```python
from build123d import *

# Parameters (mm, degrees)
SKETCH_W        = 130
SKETCH_H        = 40
SKETCH_R        = 8.5
PAD_DEPTH       = 3
SKETCH001_R     = 1.25
POCKET_DEPTH    = 5
SKETCH002_W     = 7
SKETCH002_H     = 11
POCKET001_DEPTH = 5
POCKET002_DEPTH = 5


with BuildPart() as part:
    # Sketch → Pad (new body)
    with BuildSketch(Plane.XY):
        with Locations((65, 20)):
            Rectangle(SKETCH_W, SKETCH_H)
        with Locations((40, 27.5)):
            Circle(SKETCH_R, mode=Mode.SUBTRACT)
        with Locations((90, 27.5)):
            Circle(SKETCH_R, mode=Mode.SUBTRACT)
        with Locations((15, 27.5)):
            Circle(SKETCH_R, mode=Mode.SUBTRACT)
        with Locations((115, 27.5)):
            Circle(SKETCH_R, mode=Mode.SUBTRACT)
    extrude(amount=PAD_DEPTH)

    # Sketch001 (on Face10 of Pad) → Pocket (cut)
    with BuildSketch(Plane.XY.offset(3)):
        with Locations((7, 35)):
            Circle(SKETCH001_R)
        with Locations((23, 35)):
            Circle(SKETCH001_R)
        with Locations((23, 5)):
            Circle(SKETCH001_R)
        with Locations((7, 5)):
            Circle(SKETCH001_R)
        with Locations((107, 35)):
            Circle(SKETCH001_R)
        with Locations((123, 35)):
            Circle(SKETCH001_R)
        with Locations((123, 5)):
            Circle(SKETCH001_R)
        with Locations((107, 5)):
            Circle(SKETCH001_R)
        with Locations((57, 35)):
            Circle(SKETCH001_R)
        with Locations((73, 35)):
            Circle(SKETCH001_R)
        with Locations((57, 5)):
            Circle(SKETCH001_R)
        with Locations((73, 5)):
            Circle(SKETCH001_R)
        with Locations((32, 35)):
            Circle(SKETCH001_R)
        with Locations((48, 35)):
            Circle(SKETCH001_R)
        with Locations((32, 5)):
            Circle(SKETCH001_R)
        with Locations((48, 5)):
            Circle(SKETCH001_R)
        with Locations((82, 35)):
            Circle(SKETCH001_R)
        with Locations((98, 35)):
            Circle(SKETCH001_R)
        with Locations((98, 5)):
            Circle(SKETCH001_R)
        with Locations((82, 5)):
            Circle(SKETCH001_R)
    extrude(amount=-POCKET_DEPTH, mode=Mode.SUBTRACT)

    # Sketch002 (on Face5 of Pocket) → Pocket001 (cut)
    with BuildSketch(Plane.XY.offset(3)):
        with Locations((74.5, 21.5)):
            Rectangle(SKETCH002_W, SKETCH002_H)
        with Locations((55.5, 21.5)):
            Rectangle(SKETCH002_W, SKETCH002_H)
    extrude(amount=-POCKET001_DEPTH, mode=Mode.SUBTRACT)

    # Sketch003 (on Face5 of Pocket001) → Pocket002 (cut)
    with BuildSketch(Plane.XY.offset(3)):
        with BuildLine():
            ThreePointArc((3, 40), (0.87868, 39.12132), (0, 37))
            Line((0, 37), (-3, 37))
            Line((-3, 43), (-3, 37))
            Line((3, 43), (-3, 43))
            Line((3, 40), (3, 43))
        make_face()
        with BuildLine():
            ThreePointArc((0, 3), (0.87868, 0.87868), (3, 0))
            Line((3, 0), (3, -3))
            Line((3, -3), (-3, -3))
            Line((-3, -3), (-3, 3))
            Line((0, 3), (-3, 3))
        make_face()
        with BuildLine():
            ThreePointArc((127, 0), (129.12132, 0.87868), (130, 3))
            Line((130, 3), (133, 3))
            Line((133, 3), (133, -3))
            Line((127, -3), (133, -3))
            Line((127, 0), (127, -3))
        make_face()
        with BuildLine():
            ThreePointArc((130, 37), (129.12132, 39.12132), (127, 40))
            Line((127, 40), (127, 43))
            Line((127, 43), (133, 43))
            Line((133, 37), (133, 43))
            Line((130, 37), (133, 37))
        make_face()
    extrude(amount=-POCKET002_DEPTH, mode=Mode.SUBTRACT)


solid = part.part
```
Input: part model. Units: mm. Frame: model coordinates. Coordinates: 2 decimals unless noted, no trailing zeros. Order: outer loops, then holes, each group sorted by start corner. A loop starts at its lowest first (then second) coordinate and runs counter-clockwise, first axis right, second up. Notation, with made-up numbers: (26, 50.5) - (41, 50.5) arc R29 ccw to (41, 88.5) - close; hole circle Ø3 at (23.5, -17). An arc over 180 degrees is marked (long way). Put each result on its own line as item: value.
1. Cut plane D-D on z = 1.5. State how many separate pieces and enclosed holes the cut face has, then the cut area to 3 significant figures.
Report:
separate pieces: 1
enclosed holes: 26
area: 4,030 mm2
2. Line query: line 1 along Y through (x, z) = (73, 2.15); line 2 along X through (y, z) = (17, 1.6); line 3 along X through (y, z) = (29.5, 0.4). Output: solid intervals per line, ascending.
Report:
line 1: y = 0 to 3.75, 6.25 to 16, 27 to 33.75, 36.25 to 40
line 2: x = 0 to 52, 59 to 71, 78 to 130
line 3: x = 0 to 6.74, 23.26 to 31.74, 48.26 to 81.74, 98.26 to 106.74, 123.26 to 130
3. Contact query for flat-ended pins moving along their axis: pin 1 Ø1 at (x, y) = (26, 5.5) entering from -Z; pin 2 Ø1.5 at (x, y) = (73, 5) entering from -Z. Output: stop coordinate, or through.
Report:
pin 1: stops at z = 0
pin 2: passes through
4. Cut plane B-B on y = 23.5. Return the cut outline in (x, z), then the cut area to 3 significant figures.
Report:
outline: (0, 0) - (7.5, 0) - (7.5, 3) - (0, 3) - close; (22.5, 0) - (32.5, 0) - (32.5, 3) - (22.5, 3) - close; (47.5, 0) - (52, 0) - (52, 3) - (47.5, 3) - close; (59, 0) - (71, 0) - (71, 3) - (59, 3) - close; (78, 0) - (82.5, 0) - (82.5, 3) - (78, 3) - close; (97.5, 0) - (107.5, 0) - (107.5, 3) - (97.5, 3) - close; (122.5, 0) - (130, 0) - (130, 3) - (122.5, 3) - close
area: 168 mm2
5. Draft query along X for faces 1 (the face through (47.73, 33.78, 1.52)), 2 (the face through (81.51, 27.87, 1.48)), 3 (the face through (64, 0, 1)), 4 (the face through (129.1, 0.86, 1.52)). Return one class per face: pulls with the +X half, pulls with the -X half, needs draft (parallel to the pull), parting line crosses it, or undercut.
Report:
face 1: undercut
face 2: undercut
face 3: needs draft
face 4: pulls with the +X half
6. Cut plane C-C on x = 44. Return the cut outline in (y, z).
Report:
outline: (0, 0) - (20, 0) - (20, 3) - (0, 3) - close; (35, 0) - (40, 0) - (40, 3) - (35, 3) - close
7. Cut plane A-A on x = 15. Return the cut outline in (y, z), then the cut area to 3 significant figures.
Report:
outline: (0, 0) - (19, 0) - (19, 3) - (0, 3) - close; (36, 0) - (40, 0) - (40, 3) - (36, 3) - close
area: 69.0 mm2
